Source: CAD feature listing. Evaluate the final solid. Frame: model axes, mm. A direction names the side the tool comes from. Round coordinates to 2 decimals unless told otherwise and drop trailing zeros. Write each loop counter-clockwise with the first axis right and the second up, starting at its lowest first coordinate (ties: lowest second). Pieces come first, ordered by that corner, then holes. Notation, with made-up numbers: (40, 48) -> (59, 48) arc R12 ccw to (59, 66) -> close; hole circle Ø2 at (40, -18.5). An arc over 180 degrees is marked (long way). Put each result on its own line as item: value.
Autodesk Inventor part; units mm, degrees
ref_plane "YZ Plane" through (0, 0, 0) normal (1, 0, 0) x (0, 1, 0)
ref_plane "XZ Plane" through (0, 0, 0) normal (0, 1, 0) x (-1, 0, 0)
ref_plane "XY Plane" through (0, 0, 0) normal (0, 0, 1) x (1, 0, 0)
sketch "Sketch1" plane through (0, 0, 0) normal (0, 1, 0) x (-1, 0, 0)
  line L0 (0, 0) -> (22, 0)
  line L1 (22, 0) -> (22, -12)
  line L2 (22, -12) -> (0, -12)
  line L3 (0, -12) -> (0, 0)
  dimension "d0" = 22
  dimension "d1" = 12
extrude "Extrusion1" add sketch "Sketch1" along normal blind 15
sketch "Sketch2" plane through (0, 15, 0) normal (0, 1, 0) x (1, 0, 0)
  line L0 (-27, 0) -> (5, 0)
  line L1 (5, 0) -> (5, 12)
  line L2 (5, 12) -> (-27, 12)
  line L3 (-27, 12) -> (-27, 0)
  line L4 (-22, 12) -> (-22, 0)
  line L5 (0, 0) -> (0, 12)
  point P0 (-22, 6)
  dimension "d4" = 5
  dimension "d5" = 5
extrude "Extrusion2" add sketch "Sketch2" along normal blind 2
sketch "Sketch3" plane through (0, 17, 0) normal (0, 1, 0) x (1, 0, 0)
  line L0 (-22, 0) -> (0, 0)
  line L1 (5, 12) -> (-27, 12)
  line L2 (-22, 0) -> (0, 0)
  line L3 (0, 0) -> (0, 12)
  line L4 (0, 12) -> (-22, 12)
  line L5 (-22, 12) -> (-22, 0)
  line L6 (0, 0) -> (0, 12)
extrude "Extrusion3" add sketch "Sketch3" along normal blind 4
sketch "Sketch4" plane through (0, 21, 0) normal (0, 1, 0) x (1, 0, 0)
  circle A0 centre (-16, 6) radius 6
  line L0 (-22, 12) -> (-22, 0)
  line L1 (0, 12) -> (-22, 12)
  point P0 (0, 0)
  dimension "d10" = 12
extrude "Extrusion4" add sketch "Sketch4" along normal blind 4 contours A0
sketch "Sketch5" plane through (-16, 25, -6) normal (0, 1, 0) x (1, 0, 0)
  circle A0 centre (0, 0) radius 2.5
  circle A1 centre (0, 0) radius 6
  point P0 (16, -6)
  dimension "d13" = 5
extrude "Extrusion5" add sketch "Sketch5" along normal blind 3 contours A0
sketch "Sketch6" plane through (0, 17, 0) normal (0, 1, 0) x (1, 0, 0)
  circle A0 centre (3, 6) radius 1
  circle A1 centre (-25, 6) radius 1
  line L0 (-27, 0) -> (-22, 0)
  line L1 (0, 0) -> (5, 0)
  line L2 (-27, 12) -> (-27, 0)
  point P0 (-24.5, 0)
  point P1 (2.5, 0)
  dimension "d16" = 2
  dimension "d17" = 2
  dimension "d18" = 6
  dimension "d19" = 6
  dimension "d20" = 28
  dimension "d21" = 2
extrude "Extrusion6" cut sketch "Sketch6" against normal through all
properties part number "SG-90-Servo"
Q1. Draft query along Z for faces 5 (the cylindrical face through (-10.46, 22.97, -8.3)), 6 (the cylindrical face through (-25, 16, -7)), 7 (the flat face through (-21, 21, -11)), 8 (the flat face through (-11, 10, -12)). Return one class per face: +Z half, -Z half, draft (parallel to the pull), parting line (faces both ways), or undercut.
Ans:
face 5: parting line
face 6: undercut
face 7: draft
face 8: -Z half
Q2. Reachability of faces 1 (the flat face through (-22, 7, -6)), 2 (the flat face through (0, 19, -6)), 3 (the flat face through (0, 7, -6)), 4 (the flat face through (-22, 19, -6)) from +Z, -Z, +X, -X, +Y, -Y: full face, straight path, thin tool, end or side. Return the list, or none.
Ans:
face 1: +Z, -Z, -X, -Y
face 2: +Z, -Z, +X, +Y
face 3: +Z, -Z, +X, -Y
face 4: +Z, -Z, -X, +Y
Q3. Cut plane C-C on z = -4.25. Output: boundary loops of the cut face in (x, y), and give its area (3 significant figures).
Ans:
outline: (-27, 15) -> (-22, 15) -> (-22, 0) -> (0, 0) -> (0, 15) -> (5, 15) -> (5, 17) -> (0, 17) -> (0, 21) -> (-10.26, 21) -> (-10.26, 25) -> (-14.21, 25) -> (-14.21, 28) -> (-17.79, 28) -> (-17.79, 25) -> (-21.74, 25) -> (-21.74, 21) -> (-22, 21) -> (-22, 17) -> (-27, 17) -> close
area: 539 mm^2
Q4. Cut plane A-A on x = -25. Output: boundary loops of the cut face in (y, z).
Ans:
outline: (15, -12) -> (17, -12) -> (17, -7) -> (15, -7) -> close; (15, -5) -> (17, -5) -> (17, 0) -> (15, 0) -> close
Q5. Cut plane D-D on x = -13. Output: boundary loops of the cut face in (y, z), and give its area (3 significant figures).
Ans:
outline: (0, -12) -> (21, -12) -> (21, -11.2) -> (25, -11.2) -> (25, -0.8) -> (21, -0.8) -> (21, 0) -> (0, 0) -> close
area: 294 mm^2
Q6. Material intervals for line 1 (X direction, y = 15.55, z = -6); line 2 (Z direction, x = 3, y = 16.2); line 3 (Y direction, x = -0.5, z = -11), sorted ascending. Write a range as [from, to].
Ans:
line 1: x = [-27, -26], [-24, 2], [4, 5]
line 2: z = [-12, -7], [-5, 0]
line 3: y = [0, 21]
Q7. Pin query (flat end, axial travel): pin 1 (2.5 mm diameter, centred on x = -25, z = -6, fed in from +Y); pin 2 (6 mm diameter, centred on y = 3.5, z = -10.5, fed in from +X); pin 3 (1.2 mm diameter, centred on y = 19.5, z = -7, fed in from -X); pin 4 (1.2 mm diameter, centred on x = 3, z = -6, fed in from +Y). Return the tip coordinate at first contact, or that it passes through.
Ans:
pin 1: stops at y = 17
pin 2: stops at x = 0
pin 3: stops at x = -22
pin 4: passes through
Q8. Cut plane B-B on y = 25.5. Output: boundary loops of the cut face in (x, z).
Ans:
outline: circle Ø5 at (-16, -6)
